```python
from build123d import *

# Parameters (mm, degrees)
SKETCH1_W           = 36
SKETCH1_H           = 19
BOSS_EXTRUDE1_DEPTH = 10
SKETCH2_W           = 24
SKETCH2_H           = 13
CUT_EXTRUDE1_DEPTH  = 10
SKETCH3_W           = 44
SKETCH3_H           = 33.5
BOSS_EXTRUDE2_DEPTH = 22
CUT_EXTRUDE2_REACH  = 58.926
CUT_EXTRUDE3_REACH  = 58.926
CUT_EXTRUDE4_DEPTH  = 54.124852941
CUT_EXTRUDE6_DEPTH  = 54.124852941
CUT_EXTRUDE7_DEPTH  = 54.124852941
SKETCH12_R          = 2
BOSS_EXTRUDE3_DEPTH = 2.2
BOSS_EXTRUDE3_TAPER = 1
CUT_EXTRUDE8_REACH  = 40.809
SKETCH13_W          = 24
SKETCH13_H          = 13
FILLET1_R           = 2
FILLET2_R           = 1
FILLET4_SIZE        = 2
FILLET4_SIZE_2      = 5
FILLET5_R           = 1.3


with BuildPart() as part:
    # Sketch1 → Boss-Extrude1 (new body)
    with BuildSketch(Plane(origin=(0, 0, 0), x_dir=(1, 0, 0), z_dir=(0, 1, 0))):
        Rectangle(SKETCH1_W, SKETCH1_H)
    extrude(amount=BOSS_EXTRUDE1_DEPTH)

    # Sketch2 → Cut-Extrude1 (cut)
    with BuildSketch(Plane(origin=(0, 10, 0), x_dir=(1, 0, 0), z_dir=(0, 1, 0))):
        Rectangle(SKETCH2_W, SKETCH2_H)
    extrude(amount=-CUT_EXTRUDE1_DEPTH, mode=Mode.SUBTRACT)

    # Sketch3 → Boss-Extrude2 (add)
    with BuildSketch(Plane(origin=(0, 10, 0), x_dir=(1, 0, 0), z_dir=(0, 1, 0))):
        with Locations((4, 0)):
            Rectangle(SKETCH3_W, SKETCH3_H)
    extrude(amount=BOSS_EXTRUDE2_DEPTH)

    # Sketch5 → Cut-Extrude2 (cut, up to next)
    with BuildSketch(Plane.ZY.offset(18), mode=Mode.PRIVATE) as cut_extrude2_sk1:
        Polygon((-14.55, 32), (14.55, 32), (14.55, 15.735533906), (11.014466094, 12.2), (-11.014466094, 12.2), (-14.55, 15.735533906), align=None)
    cut_extrude2_tool1 = extrude(cut_extrude2_sk1.sketch, amount=-CUT_EXTRUDE2_REACH, mode=Mode.PRIVATE) & part.part
    add(cut_extrude2_tool1.solids().sort_by_distance((-18, 22.293405, 0))[0], mode=Mode.SUBTRACT)

    # Sketch7 → Cut-Extrude3 (cut, up to next)
    with BuildSketch(Plane.ZY.offset(18), mode=Mode.PRIVATE) as cut_extrude3_sk1:
        Polygon((-16.75, 14.824264069), (-11.925735931, 10), (-16.75, 10), align=None)
    cut_extrude3_tool1 = extrude(cut_extrude3_sk1.sketch, amount=-CUT_EXTRUDE3_REACH, mode=Mode.PRIVATE) & part.part
    # Sketch7 → Cut-Extrude3 (cut, up to next)
    with BuildSketch(Plane.ZY.offset(18), mode=Mode.PRIVATE) as cut_extrude3_sk2:
        Polygon((16.75, 14.824264069), (11.925735931, 10), (16.75, 10), align=None)
    cut_extrude3_tool2 = extrude(cut_extrude3_sk2.sketch, amount=-CUT_EXTRUDE3_REACH, mode=Mode.PRIVATE) & part.part
    add(cut_extrude3_tool1.solids().sort_by_distance((-18, 11.608088, -15.141912))[0], mode=Mode.SUBTRACT)
    add(cut_extrude3_tool2.solids().sort_by_distance((-18, 11.608088, 15.141912))[0], mode=Mode.SUBTRACT)

    # Sketch9 → Cut-Extrude4 (cut, through all)
    with BuildSketch(Plane.XY.offset(16.75)):
        with BuildLine():
            Line((12.7, 23.824264069), (12.7, 16.824264069))
            ThreePointArc((12.7, 16.824264069), (12.407106781, 16.117157288), (11.7, 15.824264069))
            Line((11.7, 15.824264069), (0.501407823, 15.824264069))
            ThreePointArc((0.501407823, 15.824264069), (-0.440387617, 16.488077587), (-0.131829968, 17.598221368))
            Line((-0.131829968, 17.598221368), (8.423725588, 24.598221368))
            ThreePointArc((8.423725588, 24.598221368), (8.720776897, 24.766059508), (9.056963378, 24.824264069))
            Line((9.056963378, 24.824264069), (11.7, 24.824264069))
            ThreePointArc((11.7, 24.824264069), (12.407106781, 24.53137085), (12.7, 23.824264069))
        make_face()
    extrude(amount=-CUT_EXTRUDE4_DEPTH, mode=Mode.SUBTRACT)

    # Sketch10 → Cut-Extrude6 (cut, through all)
    with BuildSketch(Plane.XY.offset(16.75)):
        with BuildLine():
            Line((-18, 10.098548576), (4.662823879, 28.640859022))
            ThreePointArc((4.662823879, 28.640859022), (7.299328616, 30.193246078), (10.281806361, 30.875806919))
            Line((10.281806361, 30.875806919), (26, 32))
            Line((26, 32), (-18, 32))
            Line((-18, 32), (-18, 10.098548576))
        make_face()
    extrude(amount=-CUT_EXTRUDE6_DEPTH, mode=Mode.SUBTRACT)

    # Sketch11 → Cut-Extrude7 (cut, through all)
    with BuildSketch(Plane.XY.offset(16.75)):
        with BuildLine():
            Line((18, 10), (18, 22.653857453))
            ThreePointArc((18, 22.653857453), (18.292893219, 23.360964234), (19, 23.653857453))
            Line((19, 23.653857453), (21.567861559, 23.653857453))
            ThreePointArc((21.567861559, 23.653857453), (26.035822704, 27.594752604), (21.71203996, 31.693317495))
            Line((21.71203996, 31.693317495), (18, 31.427825814))
            Line((18, 31.427825814), (18, 34.061365202))
            Line((18, 34.061365202), (30.208332635, 34.9345268))
            Line((30.208332635, 34.9345268), (29.247958423, 10))
            Line((29.247958423, 10), (18, 10))
        make_face()
    extrude(amount=-CUT_EXTRUDE7_DEPTH, mode=Mode.SUBTRACT)

    # Sketch12 → Boss-Extrude3 (add)
    with BuildSketch(Plane.XY.offset(16.75)):
        with Locations((22, 27.667130408)):
            Circle(SKETCH12_R)
    boss_extrude3 = extrude(amount=BOSS_EXTRUDE3_DEPTH, taper=BOSS_EXTRUDE3_TAPER)

    # Mirror1: Boss-Extrude3 across plane
    add(boss_extrude3.mirror(Plane.XY))

    # Sketch13 → Cut-Extrude8 (cut, up to next)
    with BuildSketch(Plane.XZ.offset(-10), mode=Mode.PRIVATE) as cut_extrude8_sk1:
        Rectangle(SKETCH13_W, SKETCH13_H)
    cut_extrude8_tool1 = extrude(cut_extrude8_sk1.sketch, amount=-CUT_EXTRUDE8_REACH, mode=Mode.PRIVATE) & part.part
    add(cut_extrude8_tool1.solids().sort_by_distance((0, 10, 0))[0], mode=Mode.SUBTRACT)

    # Fillet1
    fillet1_edges = [part.edges().sort_by_distance(p)[0] for p in [
        (-18, 0, 0),
        (18, 0, 0),
    ]]
    fillet(fillet1_edges, radius=FILLET1_R)

    # Fillet2
    fillet2_edges = [part.edges().sort_by_distance(p)[0] for p in [
        (2.887937246, 14.824264069, -16.75),
        (2.887937246, 14.824264069, 16.75),
        (0, 10, -11.925735931),
        (0, 10, 11.925735931),
    ]]
    fillet(fillet2_edges, radius=FILLET2_R)

    # Fillet4
    # a fillet whose section is not a circle: 5, 2 mm, written as the material it takes off along each edge
    with BuildSketch(Plane(origin=(18, 12.2, 23.514466094), x_dir=(0, -1, 0), z_dir=(0, 0, -1))) as fillet4_piece_1_section:
        with BuildLine():
            Bezier((FILLET4_SIZE, 0), (0, 0), (0, FILLET4_SIZE_2), weights=[1, 0.707106781, 1])
            Line((0, FILLET4_SIZE_2), (0, 0))
            Line((0, 0), (FILLET4_SIZE, 0))
        make_face()
    fillet4_piece_1 = extrude(amount=47.028932188, mode=Mode.PRIVATE)
    fillet4_piece_1 = split(fillet4_piece_1, bisect_by=Plane(origin=(18, 18.45, 17.264466094), z_dir=(0, 0.7071067811865465, -0.7071067811865486)), keep=Keep.TOP, mode=Mode.PRIVATE)
    fillet4_piece_1 = split(fillet4_piece_1, bisect_by=Plane(origin=(18, -5.064466094, 6.25), z_dir=(0, 0.7071067811865478, 0.7071067811865474)), keep=Keep.TOP, mode=Mode.PRIVATE)
    add(fillet4_piece_1, mode=Mode.SUBTRACT)

    # Fillet5
    fillet5_edges = [part.edges().sort_by_distance(p)[0] for p in [
        (-15.43155937, 12.2, 0),
    ]]
    fillet(fillet5_edges, radius=FILLET5_R)


solid = part.part
```
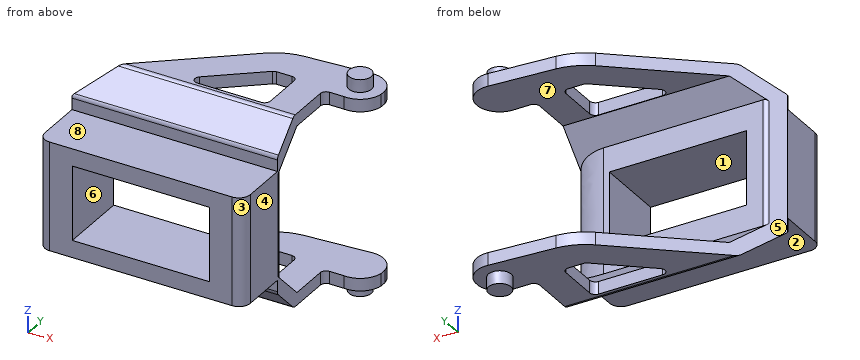
Can you work these out from the model? Positions are in its coordinate system, mm. Face numbers are marked on the shaded views. A direction names the side the tool comes from. Coordinates: 2 decimals unless noted, no trailing zeros. Loops run counter-clockwise (first coordinate to the right, second up) from the corner with the lowest first, then second, coordinate; pieces in that order, holes last. Notation, with made-up numbers: (47, -16) - (99, -16) arc R13 ccw to (99, 5) - close; hole circle Ø10 at (64.5, 87.25). An arc over 180 degrees is marked (long way). Use a Markdown table: item, result.
Item 1: Will these pins go through, and if not, where does the flat tip stop? pin 1 (0.7 mm diameter, centred on x = 7.5, z = -16, fed in from +Y); pin 2 (11 mm diameter, centred on x = -1.5, y = 7.5, fed in from -Z); pin 3 (0.6 mm diameter, centred on x = 5, z = -10, fed in from -Y); pin 4 (5 mm diameter, centred on x = -1.5, y = 27.5, fed in from -Z).
Numbers:
| item | result |
|---|---|
| pin 1 | stops at y = 30.39 |
| pin 2 | stops at z = -14.93 |
| pin 3 | stops at y = 10 |
| pin 4 | passes through |
Item 2: For the marked faces 4, 5, 6, 7 and 8, which set-ups out of +Z, -Z, +X, -X, +Y, -Y let a thin tool reach every point of the face, with its end or its side?
Numbers:
| item | result |
|---|---|
| face 4 | +Z, -Z, +X, -Y |
| face 5 | +Z, -Z, -X, +Y |
| face 6 | +Y, -Y |
| face 7 | +X, -X, +Y |
| face 8 | +Z, +X, -X, -Y |
Item 3: I want a section at A-A on y = 9. Please give me the cut outline in (x, z).
Numbers:
| item | result |
|---|---|
| outline | (-18, -9.5) - (18, -9.5) - (18, 9.5) - (-18, 9.5) - close; hole (-12, -6.5) - (12, -6.5) - (12, 6.5) - (-12, 6.5) - close |
Item 4: If I drill on probe 1 along Z at (x, y) = (15, 25); probe 2 along X at (y, z) = (2.5, 3.5); probe 3 along Y at (x, z) = (-2, -11), over which ranges is the centre line in solid material (lowest first)? Write a range as from..to.
Numbers:
| item | result |
|---|---|
| probe 1 | z = -16.75..-14.55, 14.55..16.75 |
| probe 2 | x = -18..-12, 12..18 |
| probe 3 | y = 10..12.2 |
Item 5: We'd pull the mould along X, two halves only. Please class the marked faces 1, 2 and 3: released by +X, released by -X, zero draft, split by the parting line, or undercut.
Numbers:
| item | result |
|---|---|
| face 1 | undercut |
| face 2 | zero draft |
| face 3 | released by +X |
Item 6: I want a section at C-C on y = 18.5. Please give me the cut outline in (x, z).
Numbers:
| item | result |
|---|---|
| outline | (-7.73, -16.75) - (0.97, -16.75) - (0.97, -14.55) - (-7.73, -14.55) - close; (-7.73, 14.55) - (0.97, 14.55) - (0.97, 16.75) - (-7.73, 16.75) - close; (12.7, -16.75) - (18, -16.75) - (18, -14.55) - (12.7, -14.55) - close; (12.7, 14.55) - (18, 14.55) - (18, 16.75) - (12.7, 16.75) - close |
Item 7: I want a section at D-D on z = 13. Please give me the cut outline in (x, y).
Numbers:
| item | result |
|---|---|
| outline | (-16.81, 11.07) - (18, 11.07) - (18, 14.19) - (-13, 14.19) - close |
Item 8: I want a section at B-B on x = -10.5. Please give me the cut outline in (y, z).
Numbers:
| item | result |
|---|---|
| outline | (0, -9.5) - (10, -9.5) - (10, -11.51) arc R1 ccw to (10.29, -12.22) - (14.53, -16.46) arc R1 ccw to (15.24, -16.75) - (16.23, -16.75) - (16.23, -14.55) - (15.74, -14.55) - (12.2, -11.01) - (12.2, -6.5) - (0, -6.5) - close; (0, 6.5) - (12.2, 6.5) - (12.2, 11.01) - (15.74, 14.55) - (16.23, 14.55) - (16.23, 16.75) - (15.24, 16.75) arc R1 ccw to (14.53, 16.46) - (10.29, 12.22) arc R1 ccw to (10, 11.51) - (10, 9.5) - (0, 9.5) - close |
